from build123d import *

# Parameters (mm, degrees)
F1_DEPTH = 34.925


with BuildPart() as f1:
    # F0 (on Top) → F1 (new body)
    with BuildSketch(Plane.XY):
        with BuildLine():
            Line((1200.15, 0), (127, 0))
            Line((127, 0), (0, -127))
            Line((0, -127), (0, -1200.15))
            Line((0, -1200.15), (600.075, -1200.15))
            ThreePointArc((600.075, -1200.15), (775.832898, -775.832898), (1200.15, -600.075))
            Line((1200.15, -600.075), (1200.15, 0))
        make_face()
    extrude(amount=-F1_DEPTH)


solid = f1.part
Can you work these out from the model? Positions are in its coordinate system, mm. Coordinates: 2 decimals unless noted, no trailing zeros. Write each loop counter-clockwise with the first axis right and the second up, starting at its lowest first coordinate (ties: lowest second). Pieces come first, ordered by that corner, then holes. Notation, with made-up numbers: (56.5, 77.25) -> (98.5, 77.25) arc R22 cw to (98.5, 107.25) -> close; hole circle Ø1 at (24.25, -25). An arc over 180 degrees is marked (long way). Write each question's results on one line, items separated by ' | '. Start each with the question number.
Item 1: If we section it at A-A, the plane z = -15.5: Write out the boundary of the cut face in (x, y) (3 decimals).
Item 2: Please list where these lines run through material, in increasing order: probe 1 along X at (y, z) = (-838, -23); probe 2 along X at (y, z) = (-921, -10.5); probe 3 along Y at (x, z) = (852.5, -22.5).
Item 3: If we section it at C-C, the plane x = 1002: Write out the boundary of the cut face in (y, z) (3 decimals).
Item 4: If we section it at B-B, the plane y = -858: Write out the boundary of the cut face in (x, z) (3 decimals).
Item 5: I'm going to push flat-ended pins straight in: P1, Ø3, axis at x = 778, z = -21.5, coming from the -Y side; P2, Ø2, axis at y = -981, z = -25.5, coming from the +X side. Where does each tip first touch, or does it pass through?
Answer block:
1) outline: (0, -1200.15) -> (600.075, -1200.15) arc R600.075 cw to (1200.15, -600.075) -> (1200.15, 0) -> (127, 0) -> (0, -127) -> close
2) probe 1: 0 to 721.68 | probe 2: 0 to 668.96 | probe 3: -711.04 to 0
3) outline: (-633.734, -34.925) -> (0, -34.925) -> (0, 0) -> (-633.734, 0) -> close
4) outline: (0, -34.925) -> (707.176, -34.925) -> (707.176, 0) -> (0, 0) -> close
5) P1: y = -775.17 | P2: x = 641.92
